from build123d import *
from build123d.topology import SkipClean

# Parameters (mm, degrees)
BOSS_EXTRUDE1_DEPTH = 7.5
BOSS_EXTRUDE3_START = -7.5
SKETCH1_7_R         = 7.35
BOSS_EXTRUDE3_DEPTH = 50


with BuildPart() as part:
    # Sketch1 → Boss-Extrude1 (new, symmetric)
    with BuildSketch(Plane(origin=(0, 0, 0), x_dir=(1, 0, 0), z_dir=(0, 1, 0))):
        with BuildLine():
            ThreePointArc((6.122564101, 4.581600452), (5.584294246, 5.185414455), (4.982932131, 5.726422213))
            Line((4.982932131, 5.726422213), (3.28457771, 4.028067792))
            ThreePointArc((3.28457771, 4.028067792), (2.292289605, 4.584151566), (1.199538666, 4.9))
            Line((1.199538666, 4.9), (1.199538666, 7.303634322))
            ThreePointArc((1.199538666, 7.303634322), (0.391963425, 7.349981033), (-0.415814059, 7.307304058))
            Line((-0.415814059, 7.307304058), (-0.415814059, 4.905468202))
            ThreePointArc((-0.415814059, 4.905468202), (-1.510678314, 4.597025162), (-2.506708483, 4.047672132))
            Line((-2.506708483, 4.047672132), (-4.206334611, 5.747298261))
            ThreePointArc((-4.206334611, 5.747298261), (-4.810148615, 5.209028406), (-5.351156372, 4.60766629))
            Line((-5.351156372, 4.60766629), (-3.652801952, 2.909311869))
            ThreePointArc((-3.652801952, 2.909311869), (-4.208885725, 1.917023764), (-4.524734159, 0.824272826))
            Line((-4.524734159, 0.824272826), (-6.928368481, 0.824272826))
            ThreePointArc((-6.928368481, 0.824272826), (-6.974715193, 0.016697585), (-6.932038217, -0.791079899))
            Line((-6.932038217, -0.791079899), (-4.530202362, -0.791079899))
            ThreePointArc((-4.530202362, -0.791079899), (-4.221759321, -1.885944155), (-3.672406292, -2.881974323))
            Line((-3.672406292, -2.881974323), (-5.37203242, -4.581600452))
            ThreePointArc((-5.37203242, -4.581600452), (-4.833762565, -5.185414455), (-4.23240045, -5.726422213))
            Line((-4.23240045, -5.726422213), (-2.534046029, -4.028067792))
            ThreePointArc((-2.534046029, -4.028067792), (-1.541757924, -4.584151566), (-0.449006985, -4.9))
            Line((-0.449006985, -4.9), (-0.449006985, -7.303634322))
            ThreePointArc((-0.449006985, -7.303634322), (0.358568256, -7.349981033), (1.16634574, -7.307304058))
            Line((1.16634574, -7.307304058), (1.16634574, -4.905468202))
            ThreePointArc((1.16634574, -4.905468202), (2.261209995, -4.597025162), (3.257240164, -4.047672132))
            Line((3.257240164, -4.047672132), (4.956866292, -5.747298261))
            ThreePointArc((4.956866292, -5.747298261), (5.560680296, -5.209028406), (6.101688053, -4.60766629))
            Line((6.101688053, -4.60766629), (4.403333633, -2.909311869))
            ThreePointArc((4.403333633, -2.909311869), (4.959417406, -1.917023764), (5.275265841, -0.824272826))
            Line((5.275265841, -0.824272826), (7.678900162, -0.824272826))
            ThreePointArc((7.678900162, -0.824272826), (7.725246874, -0.016697585), (7.682569898, 0.791079899))
            Line((7.682569898, 0.791079899), (5.280734043, 0.791079899))
            ThreePointArc((5.280734043, 0.791079899), (4.972291002, 1.885944155), (4.422937973, 2.881974323))
            Line((4.422937973, 2.881974323), (6.122564101, 4.581600452))
        make_face()
    extrude(amount=BOSS_EXTRUDE1_DEPTH, both=True)

    # Boss-Extrude2 cone 1 section (through the dimple's axis) → Boss-Extrude2 (revolve)
    with BuildSketch(Plane(origin=(0.375265841, 7.5, 0), x_dir=(0, 0, -1), z_dir=(1, 0, 0))):
        Polygon((0, 0), (7.35, 0), (0, 8.759388906), align=None)
    revolve(axis=Axis((0.375265841, 7.5, 0), (0, 1, 0)))

    # Sketch1<7> → Boss-Extrude3 (add)
    with SkipClean():  # the faces are left unmerged after this step: merging them gives an invalid solid
        with BuildSketch(Plane(origin=(0, 0, 0), x_dir=(1, 0, 0), z_dir=(0, 1, 0)).offset(BOSS_EXTRUDE3_START)):
            with Locations(Location((0.375265841, 0, 0), (0, 0, 96.178708688))):
                Circle(SKETCH1_7_R)
        extrude(amount=-BOSS_EXTRUDE3_DEPTH)


solid = part.part
Read the model definition and answer for the solid it produces. Units are mm, in the model's axes. A direction names the side the tool comes from. Round coordinates to 2 decimals unless told otherwise and drop trailing zeros. Write each loop counter-clockwise with the first axis right and the second up, starting at its lowest first coordinate (ties: lowest second). Pieces come first, ordered by that corner, then holes. Notation, with made-up numbers: M 32,-2 L 55,-2 A20 ccw 55,23 Z; hole C 22.5,26 d11. An arc over 180 degrees is marked long. Use a Markdown table: item, result.
1) Flat-ended cylindrical pins translate along their axes: pin 1 (1 mm diameter, centred on y = -23, z = 5, fed in from -X); pin 2 (2 mm diameter, centred on x = 3.5, z = 2.5, fed in from +Y); pin 3 (5 mm diameter, centred on x = 2, y = -14.5, fed in from +Z); pin 4 (2.5 mm diameter, centred on y = 3, z = -6.5, fed in from -X). Find the tip coordinate at first contact, or state that the pin passes through.
Answers follow:
| item | result |
|---|---|
| pin 1 | stops at x = -5.44 |
| pin 2 | stops at y = 12.68 |
| pin 3 | stops at z = 7.35 |
| pin 4 | stops at x = -4.77 |
2) Straight lines are drawn through the part: line 1 along X through (y, z) = (-1.5, 4.5); line 2 along Z through (x, y) = (5.5, -4.5); line 3 along Z through (x, y) = (4.5, -0.5). For each, find the intervals that lie inside material, in ascending order. Write a range as [from, to].
Answers follow:
| item | result |
|---|---|
| line 1 | x = [-5.29, -3.01], [-1.73, 2.48], [3.71, 5.99] |
| line 2 | z = [-5.27, -3.96], [-0.79, 0.82], [4.01, 5.27] |
| line 3 | z = [-5.24, -2.96], [-2.77, 2.77], [3.01, 5.29] |
3) The part is cut by section B-B (y = -14.5). Write down the section's boundary in (x, z), plus the area to 3 significant figures.
Answers follow:
| item | result |
|---|---|
| outline | C 0.38,0 d14.7 |
| area | 170 mm2 |
4) For a pull along Y with two mould halves and no side action, classify faces 5 (the flat face through (5.264, 0.105, 3.77)), 6 (the flat face through (-5, 7.5, 2)), 7 (the flat face through (0, -57.5, 0)) as pulls with the +Y half, pulls with the -Y half, needs draft (parallel to the pull), parting line crosses it, or undercut.
Answers follow:
| item | result |
|---|---|
| face 5 | undercut |
| face 6 | undercut |
| face 7 | pulls with the -Y half |
5) A tool of negligible diameter and unlimited length cuts with its end or side. For faces 1 (the flat face through (-5, 7.5, -2)), 2 (the flat face through (-3.345, 0.105, -4.886)), 3 (the cylindrical face through (-1.556, 0.105, 4.578)), 4 (the flat face through (6, 0, -0.791)), from which of +Z, -Z, +X, -X, +Y, -Y can it reach the whole face along a straight path? Write none if from no direction.
Answers follow:
| item | result |
|---|---|
| face 1 | -X |
| face 2 | -Z |
| face 3 | +Z |
| face 4 | +X |
